```python
from build123d import *

# Parameters (mm, degrees)
F1_DEPTH = 1
F2_R     = 4
F3_DEPTH = 12
F3_TAPER = 13
F4_R     = 0.7295817065
F5_DEPTH = 5


with BuildPart() as f1:
    # F0 (on Top) → F1 (new body)
    with BuildSketch(Plane.XY):
        with BuildLine():
            ThreePointArc((0, 1), (0.2928932188, 0.2928932188), (1, 0))
            Line((1, 0), (9, 0))
            ThreePointArc((9, 0), (9.7071067812, 0.2928932188), (10, 1))
            Line((10, 1), (10, 9))
            ThreePointArc((10, 9), (9.7071067812, 9.7071067812), (9, 10))
            Line((9, 10), (1, 10))
            ThreePointArc((1, 10), (0.2928932188, 9.7071067812), (0, 9))
            Line((0, 9), (0, 1))
        make_face()
    extrude(amount=F1_DEPTH)

    # F2 (on face) → F3 (join)
    with BuildSketch(Plane.XY.offset(1)):
        with Locations((5, 5)):
            Circle(F2_R)
    extrude(amount=F3_DEPTH, taper=F3_TAPER)

    # F4 (on face) → F5 (cut)
    with BuildSketch(Plane.XY.offset(13)):
        with Locations((5, 5)):
            Circle(F4_R)
    extrude(amount=-F5_DEPTH, mode=Mode.SUBTRACT)


solid = f1.part
```
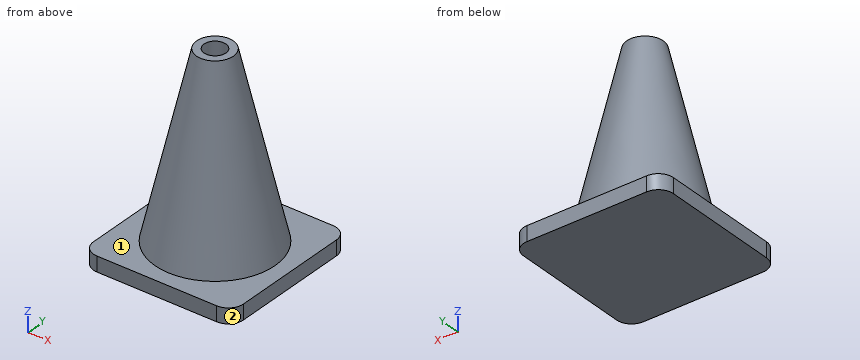
CAD build for the part. Positions are in the model's coordinates, mm. Face numbers are marked on the shaded views. A direction names the side the tool comes from. Round coordinates to 2 decimals unless told otherwise and drop trailing zeros. Write each loop counter-clockwise with the first axis right and the second up, starting at its lowest first coordinate (ties: lowest second). Pieces come first, ordered by that corner, then holes. Notation, with made-up numbers: M 49,-31 L 86,-31 A30 ccw 86,-4 Z; hole C -28,5 d10. An arc over 180 degrees is marked long. One line per question, with ' | ' between items.
1. Cut at C-C on z = 9.5. Write the cut outline in (x, y), and give its area (3 significant figures).
Working result:
outline: C 5,5 d4.08; hole C 5,5 d1.46 | area: 11.4 mm2
2. Cut at D-D on z = 1.75. Write the cut outline in (x, y).
Working result:
outline: C 5,5 d7.65
3. Which spindle directions (+Z, -Z, +X, -X, +Y, -Y) get a long thin tool onto all of the face, cutting with end or side? Do the marked faces 1 and 2. Say none if no direction does.
Working result:
face 1: +Z | face 2: +Z, -Z, +X, -Y
4. Cut at A-A on x = 5. Write the cut outline in (y, z), and give its area (3 significant figures).
Working result:
outline: M 0,0 L 10,0 L 10,1 L 9,1 L 6.23,13 L 5.73,13 L 5.73,8 L 4.27,8 L 4.27,13 L 3.77,13 L 1,1 L 0,1 Z | area: 65.5 mm2
5. Pin check, flat tips, straight feed: pin 1 Ø1.6 at (x, y) = (5.5, 5.5) entering from +Z; pin 2 Ø0.9 at (x, y) = (5, 5) entering from +Z; pin 3 Ø1 at (y, z) = (3, 3.5) entering from +X. Stop position of each tip, or through.
Working result:
pin 1: z = 13 | pin 2: z = 8 | pin 3: x = 8.11
6. Probe L1, parallel to Z at x = 9.75, y = 3.5; L2, parallel to Y at x = 5, z = 11.2; L3, parallel to X at y = 5.5, z = 12.25. List the from-to ranges inside material, lowest first. Write a range as from..to.
Working result:
L1: 0..1 | L2: 3.35..4.27, 5.73..6.65 | L3: 3.69..4.47, 5.53..6.31
